For this review, use the dimensioned drawing (mm, ordinates from the lowest corner) and the shaded views. Give positions to 0.01 mm unless a question says otherwise; leave off trailing zeros. Order: outer loops, then holes, each group sorted by start corner. A loop starts at its lowest first (then second) coordinate and runs counter-clockwise, first axis right, second up. Notation, with made-up numbers: (26.5, 1.25) -> (77.5, 1.25) arc R30 cw to (77.5, 23.25) -> close; hole circle Ø8 at (87.5, 5). An arc over 180 degrees is marked (long way). Return JSON: item names as keys, results as strings.
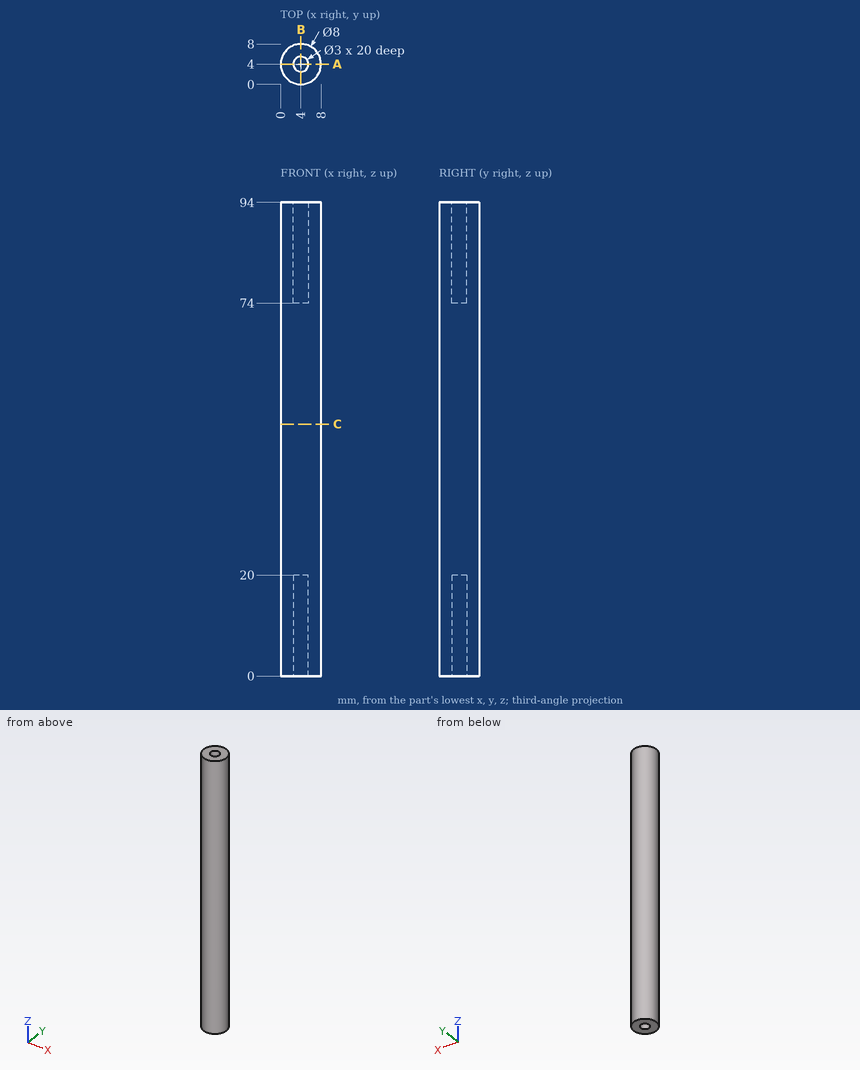
Item 1: For pin 1 (1.5 mm diameter, centred on x = 5.5, z = 16, fed in from +Y); pin 2 (1.5 mm diameter, centred on y = 6.5, z = 72.5, fed in from +X), all flat-tipped, find the tip position at first contact; note any pin that passes through.
Result set:
{"pin 1": "stops at y = 7.93", "pin 2": "stops at x = 7.6"}
Item 2: Add section C-C (z = 50). Give the boundary of the cut face in (x, y).
Result set:
{"outline": "circle Ø8 at (4, 4)"}
Item 3: Add section A-A (y = 4). Give the boundary of the cut face in (x, z).
Result set:
{"outline": "(0, 0) -> (2.5, 0) -> (2.5, 20) -> (5.5, 20) -> (5.5, 0) -> (8, 0) -> (8, 94) -> (5.5, 94) -> (5.5, 74) -> (2.5, 74) -> (2.5, 94) -> (0, 94) -> close"}
Item 4: Wall thickness on L1, parallel to Y at x = 4, z = 15.25; L2, parallel to Z at x = 3.5, y = 3; L3, parallel to X at y = 5, z = 85: over which ranges is each line inside the solid? List them lowest first. Write a range as [from, to].
Result set:
{"L1": "y = [0, 2.5], [5.5, 8]", "L2": "z = [20, 74]", "L3": "x = [0.13, 2.88], [5.12, 7.87]"}
